```python
from build123d import *

# Parameters (mm, degrees)
SKETCH1_R           = 4.25
SKETCH1_R_2         = 1.15
BOSS_EXTRUDE1_DEPTH = 5


with BuildPart() as part:
    # Sketch1 → Boss-Extrude1 (new body)
    with BuildSketch(Plane.XY):
        with BuildLine():
            Line((11.5, 46), (15, 46))
            Line((15, 46), (15, 51))
            Line((15, 51), (20, 51))
            Line((20, 51), (20, 46))
            Line((20, 46), (22, 46))
            ThreePointArc((22, 46), (26, 42), (30, 46))
            Line((30, 46), (32, 46))
            Line((32, 46), (32, 51))
            Line((32, 51), (37, 51))
            Line((37, 51), (37, 46))
            Line((37, 46), (40.5, 46))
            Line((40.5, 46), (40.5, 43))
            Line((40.5, 43), (39.4, 43))
            Line((39.4, 43), (39.4, 40.7))
            Line((39.4, 40.7), (40.5, 40.7))
            Line((40.5, 40.7), (40.5, 36))
            Line((40.5, 36), (43.5, 36))
            Line((43.5, 36), (43.5, 40.7))
            Line((43.5, 40.7), (44.6, 40.7))
            Line((44.6, 40.7), (44.6, 43))
            Line((44.6, 43), (43.5, 43))
            Line((43.5, 43), (43.5, 46))
            Line((43.5, 46), (47, 46))
            Line((47, 46), (47, 51))
            Line((47, 51), (52, 51))
            Line((52, 51), (52, 0))
            Line((52, 0), (52, -5))
            Line((52, -5), (47, -5))
            Line((47, -5), (47, 0))
            Line((47, 0), (43.5, 0))
            Line((43.5, 0), (43.5, 3))
            Line((43.5, 3), (44.6, 3))
            Line((44.6, 3), (44.6, 5.3))
            Line((44.6, 5.3), (43.5, 5.3))
            Line((43.5, 5.3), (43.5, 10))
            Line((43.5, 10), (40.5, 10))
            Line((40.5, 10), (40.5, 5.3))
            Line((40.5, 5.3), (39.4, 5.3))
            Line((39.4, 5.3), (39.4, 3))
            Line((39.4, 3), (40.5, 3))
            Line((40.5, 3), (40.5, 0))
            Line((40.5, 0), (37, 0))
            Line((37, 0), (37, -5))
            Line((37, -5), (32, -5))
            Line((32, -5), (32, 0))
            Line((32, 0), (30, 0))
            ThreePointArc((30, 0), (26, 4), (22, 0))
            Line((22, 0), (20, 0))
            Line((20, 0), (20, -5))
            Line((20, -5), (15, -5))
            Line((15, -5), (15, 0))
            Line((15, 0), (11.5, 0))
            Line((11.5, 0), (11.5, 3))
            Line((11.5, 3), (12.6, 3))
            Line((12.6, 3), (12.6, 5.3))
            Line((12.6, 5.3), (11.5, 5.3))
            Line((11.5, 5.3), (11.5, 10))
            Line((11.5, 10), (8.5, 10))
            Line((8.5, 10), (8.5, 5.3))
            Line((8.5, 5.3), (7.4, 5.3))
            Line((7.4, 5.3), (7.4, 3))
            Line((7.4, 3), (8.5, 3))
            Line((8.5, 3), (8.5, 0))
            Line((8.5, 0), (5, 0))
            Line((5, 0), (5, -5))
            Line((5, -5), (0, -5))
            Line((0, -5), (0, 0))
            Line((0, 0), (0, 51))
            Line((0, 51), (5, 51))
            Line((5, 51), (5, 46))
            Line((5, 46), (8.5, 46))
            Line((8.5, 46), (8.5, 43))
            Line((8.5, 43), (7.4, 43))
            Line((7.4, 43), (7.4, 40.7))
            Line((7.4, 40.7), (8.5, 40.7))
            Line((8.5, 40.7), (8.5, 36))
            Line((8.5, 36), (11.5, 36))
            Line((11.5, 36), (11.5, 40.7))
            Line((11.5, 40.7), (12.6, 40.7))
            Line((12.6, 40.7), (12.6, 43))
            Line((12.6, 43), (11.5, 43))
            Line((11.5, 43), (11.5, 46))
        make_face()
        with Locations((26, 15)):
            Circle(SKETCH1_R, mode=Mode.SUBTRACT)
        with Locations((26, 25)):
            Circle(SKETCH1_R_2, mode=Mode.SUBTRACT)
        with Locations((34.660254038, 20)):
            Circle(SKETCH1_R_2, mode=Mode.SUBTRACT)
        with Locations((34.660254038, 10)):
            Circle(SKETCH1_R_2, mode=Mode.SUBTRACT)
        with Locations((17.339745962, 10)):
            Circle(SKETCH1_R_2, mode=Mode.SUBTRACT)
        with Locations((17.339745962, 20)):
            Circle(SKETCH1_R_2, mode=Mode.SUBTRACT)
    extrude(amount=BOSS_EXTRUDE1_DEPTH)


solid = part.part
```
Design review of the part built by this model. Coordinates are the model's own, in mm. A direction names the side the tool comes from. Give positions to 0.01 mm unless a question says otherwise; leave off trailing zeros. Order: outer loops, then holes, each group sorted by start corner. A loop starts at its lowest first (then second) coordinate and runs counter-clockwise, first axis right, second up. Notation, with made-up numbers: (81.5, 67.25) - (113.5, 67.25) arc R25 ccw to (113.5, 104.25) - close; hole circle Ø6 at (19.25, 15.25). An arc over 180 degrees is marked (long way). Use a Markdown table: item, result. Add a question column.
(1) Add section C-C on y = -1. Give the boundary of the cut face in (x, z).
(2) Clearance check with flat-ended pins moving along their axes: P1, Ø1.8, axis at x = 7.5, z = 1.5, coming from the -Y side; P2, Ø6, axis at x = 10.5, y = 42.5, coming from the -Z side; P3, Ø1, axis at x = 38.5, z = 4, coming from the +Y side. State where each tip first meets the part, or that it passes through.
(3) Wall thickness on probe 1 along Y at (x, z) = (26, 2); probe 2 along X at (y, z) = (8.5, 1); probe 3 along Y at (x, z) = (17, 4.6): over which ranges is each line inside the solid? List them lowest first. Write a range as [from, to].
(4) Add section D-D on x = 29. Give the boundary of the cut face in (y, z).
(5) Add section B-B on x = 17. Give the boundary of the cut face in (y, z).
(6) Mouldability with a two-part tool opening along X and no side actions: class faces 1 (the face through (26, 23, 0)), 2 (the face through (47, 48, 2)) as +X half, -X half, draft (parallel to the pull), parting line (faces both ways), or undercut.
(7) Add section A-A on y = 20. Give the boundary of the cut face in (x, z), then the cut area to 3 significant figures.
(8) Machinability: for faces 3 (the face through (43.5, 8, 2)), 4 (the face through (7.4, 4, 2)), 5 (the face through (50, -5, 2)), 6 (the face through (43.5, 38, 2)), which of the approach directions +Z, -Z, +X, -X, +Y, -Y give a long, thin tool a straight path to every point of the face, cutting with its end or side? Answer none if there is none.
Report:
| question | item | result |
|---|---|---|
| 1 | outline | (0, 0) - (5, 0) - (5, 5) - (0, 5) - close; (15, 0) - (20, 0) - (20, 5) - (15, 5) - close; (32, 0) - (37, 0) - (37, 5) - (32, 5) - close; (47, 0) - (52, 0) - (52, 5) - (47, 5) - close |
| 2 | P1 | stops at y = 0 |
| 2 | P2 | stops at z = 0 |
| 2 | P3 | stops at y = 46 |
| 3 | probe 1 | y = [4, 10.75], [19.25, 23.85], [26.15, 42] |
| 3 | probe 2 | x = [0, 8.5], [11.5, 40.5], [43.5, 52] |
| 3 | probe 3 | y = [-5, 8.9], [11.1, 18.9], [21.1, 51] |
| 4 | outline | (2.65, 0) - (11.99, 0) - (11.99, 5) - (2.65, 5) - close; (18.01, 0) - (43.35, 0) - (43.35, 5) - (18.01, 5) - close |
| 5 | outline | (-5, 0) - (8.9, 0) - (8.9, 5) - (-5, 5) - close; (11.1, 0) - (18.9, 0) - (18.9, 5) - (11.1, 5) - close; (21.1, 0) - (51, 0) - (51, 5) - (21.1, 5) - close |
| 6 | face 1 | draft |
| 6 | face 2 | undercut |
| 7 | outline | (0, 0) - (16.19, 0) - (16.19, 5) - (0, 5) - close; (18.49, 0) - (33.51, 0) - (33.51, 5) - (18.49, 5) - close; (35.81, 0) - (52, 0) - (52, 5) - (35.81, 5) - close |
| 7 | area | 237 mm² |
| 8 | face 3 | +Z, -Z, -Y |
| 8 | face 4 | +Z, -Z |
| 8 | face 5 | +Z, -Z, +X, -X, -Y |
| 8 | face 6 | +Z, -Z, +Y |
